Work out the finished part from the listing and answer in its coordinate system (mm). Face numbers are marked on the shaded views. Coordinates: 2 decimals unless noted, no trailing zeros. Order: outer loops, then holes, each group sorted by start corner. A loop starts at its lowest first (then second) coordinate and runs counter-clockwise, first axis right, second up.
1. The part is cut by section D-D, the plane x = 21.5. Give the vertices of the cut face in (y, z) (3 decimals).
2. The part is cut by section C-C, the plane z = 25.4. Give the vertices of the cut face in (x, y) (3 decimals), then the cut area to 3 significant figures.
3. Find the intervals of material crossed by probe 1 along Z at (x, y) = (44.45, -14) (3 decimals); probe 2 along Z at (x, y) = (17.5, -6); probe 3 along Z at (x, y) = (40, -5), in increasing order.
4. Determine the mould class of the marked faces 1, 2, 3 and 4 for opening direction X: +X half, -X half, draft (parallel to the pull), parting line (faces both ways), or undercut.
5. The part is cut by section A-A, the plane x = 44.45. Give the vertices of the cut face in (y, z) (3 decimals), then the cut area to 3 significant figures.
6. Flat-ended cylindrical pins translate along their axes: pin 1 Ø6 at (x, y) = (23, -10.5) entering from -Z; pin 2 Ø10 at (y, z) = (-9.525, 25.4) entering from -X. Find the tip coordinate at first contact, or state that the pin passes through.
7. The part is cut by section B-B, the plane y = -14.25. Give the vertices of the cut face in (x, z) (3 decimals).
```python
from build123d import *

# Parameters (mm, degrees)
F0_W     = 88.9
F0_H     = 19.05
F1_DEPTH = 152.4
F3_D     = 12.7
F5_D     = 12.7


with BuildPart() as f1:
    # F0 (on Top) → F1 (new body)
    with BuildSketch(Plane.XY):
        with Locations((44.45, -9.525)):
            Rectangle(F0_W, F0_H)
    extrude(amount=F1_DEPTH)

    # F3 (through all)
    with Locations(Plane.XZ.offset(19.05)):
        with Locations((44.45, 123.825)):
            Hole(F3_D / 2)

    # F5 (through all)
    with Locations(Plane.YZ.offset(88.9)):
        with Locations((-9.525, 25.4)):
            Hole(F5_D / 2)


solid = f1.part
```
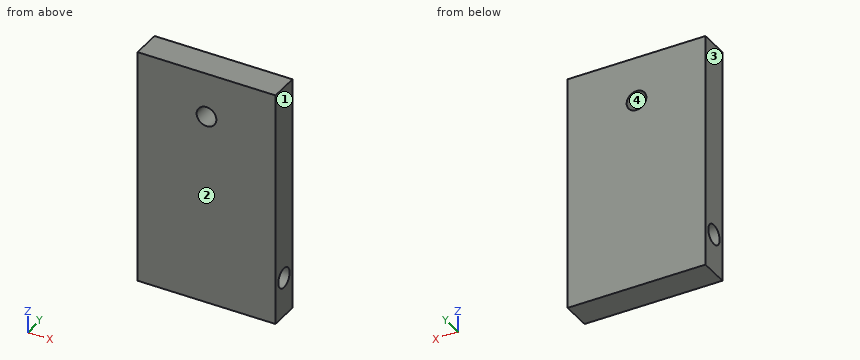
Geometry says:
1. outline: (-19.05, 0) - (0, 0) - (0, 152.4) - (-19.05, 152.4) - close; hole circle Ø12.7 at (-9.525, 25.4)
2. outline: (0, -19.05) - (88.9, -19.05) - (88.9, -15.875) - (0, -15.875) - close; (0, -3.175) - (88.9, -3.175) - (88.9, 0) - (0, 0) - close
2. area: 565 mm2
3. probe 1: z = 0 to 20.895, 29.905 to 117.475, 130.175 to 152.4
3. probe 2: z = 0 to 20.12, 30.68 to 152.4
3. probe 3: z = 0 to 20.95, 29.85 to 119.3, 128.35 to 152.4
4. face 1: +X half
4. face 2: draft
4. face 3: -X half
4. face 4: undercut
5. outline: (-19.05, 0) - (0, 0) - (0, 117.475) - (-19.05, 117.475) - close; (-19.05, 130.175) - (0, 130.175) - (0, 152.4) - (-19.05, 152.4) - close; hole circle Ø12.7 at (-9.525, 25.4)
5. area: 2,530 mm2
6. pin 1: stops at z = 0
6. pin 2: passes through
7. outline: (0, 0) - (88.9, 0) - (88.9, 21.158) - (0, 21.158) - close; (0, 29.642) - (88.9, 29.642) - (88.9, 152.4) - (0, 152.4) - close; hole circle Ø12.7 at (44.45, 123.825)
